from build123d import *

# Parameters (mm, degrees)
EXTRUDE_THIN1_DEPTH          = 123.825
F_10_CLEARANCE_HOLE1_D       = 5.334
F_3_8_0_375_DIAMETER_HOLE1_D = 9.525


with BuildPart() as part:
    # Sketch1 → Extrude-Thin1 (new, symmetric)
    with BuildSketch(Plane(origin=(0, 0, 0), x_dir=(0, 0, -1), z_dir=(1, 0, 0))):
        Polygon((-38.1, 0), (0, 0), (0, 38.1), (-6.35, 38.1), (-6.35, 6.35), (-38.1, 6.35), align=None)
    extrude(amount=EXTRUDE_THIN1_DEPTH, both=True)

    # #10 Clearance Hole1 (through all)
    with Locations(Plane(origin=(0, 6.35, 0), x_dir=(1, 0, 0), z_dir=(0, 1, 0))):
        with Locations((-114.3, -15.875), (-114.3, -28.575), (-88.9, -28.575), (-88.9, -15.875), (88.9, -15.875), (88.9, -28.575), (114.3, -28.575), (114.3, -15.875)):
            Hole(F_10_CLEARANCE_HOLE1_D / 2)

    # 3/8 (0.375) Diameter Hole1 (through all)
    with Locations(Plane.XY.offset(6.35)):
        with Locations((-95.25, 25.4), (95.25, 25.4)):
            Hole(F_3_8_0_375_DIAMETER_HOLE1_D / 2)


solid = part.part
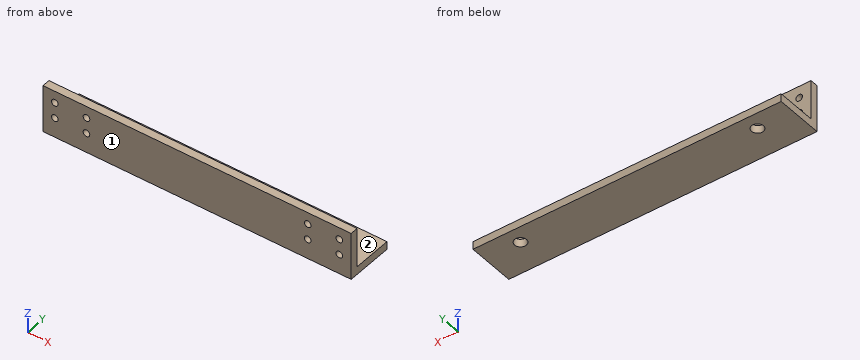
The listing builds one solid part. Answer for the finished solid, in the listing's coordinates (mm). Face numbers are marked on the shaded views. A direction names the side the tool comes from. Give positions to 0.01 mm unless a question says otherwise; leave off trailing zeros. Loops run counter-clockwise (first coordinate to the right, second up) from the corner with the lowest first, then second, coordinate; pieces in that order, holes last. Notation, with made-up numbers: (-27.75, -28) - (-9.75, -28) arc R7 ccw to (-9.75, -23) - close; hole circle Ø2 at (66, -30.75). An arc over 180 degrees is marked (long way). Write each question's results on one line, items separated by ' | '.
1. Find section B-B, the plane x = 114.3. Write down the section's boundary in (y, z).
Resolved:
outline: (0, 0) - (38.1, 0) - (38.1, 6.35) - (6.35, 6.35) - (6.35, 13.21) - (0, 13.21) - close; (0, 18.54) - (6.35, 18.54) - (6.35, 25.91) - (0, 25.91) - close; (0, 31.24) - (6.35, 31.24) - (6.35, 38.1) - (0, 38.1) - close
2. Which of the six approach directions +Z, -Z, +X, -X, +Y, -Y give full straight-line access (tool end or side, diameter ignored) to the marked faces 1 and 2?
Resolved:
face 1: +Z, -Z, +X, -X, -Y | face 2: +Z, +X, -X, +Y
3. Flat-ended cylindrical pins translate along their axes: P1, Ø16, axis at x = -51, z = 21.5, coming from the +Y side; P2, Ø15, axis at x = 95.25, y = 25.4, coming from the +Z side. Find the tip coordinate at first contact, or state that the pin passes through.
Resolved:
P1: stops at y = 6.35 | P2: stops at z = 6.35
4. Find section A-A, the plane y = 25.4. Count the separate pieces of the cut face and the enclosed holes in it, then the cut area to 3 significant figures.
Resolved:
separate pieces: 3 | enclosed holes: 0 | area: 1,450 mm^2
5. Consider probe 1 along Z at (x, y) = (88.9, 1.5); probe 2 along Z at (x, y) = (-88, 2); probe 3 along Z at (x, y) = (91, 31). Determine where each line is inside the solid, lowest interval first. Write a range as from..to.
Resolved:
probe 1: z = 0..13.21, 18.54..25.91, 31.24..38.1 | probe 2: z = 0..13.36, 18.39..26.06, 31.09..38.1 | probe 3: z = 0..6.35
6. Find section D-D, the plane x = 38. Write down the section's boundary in (y, z).
Resolved:
outline: (0, 0) - (38.1, 0) - (38.1, 6.35) - (6.35, 6.35) - (6.35, 38.1) - (0, 38.1) - close
